The listing builds one solid part. Answer for the finished solid, in the listing's coordinates (mm). A direction names the side the tool comes from. Give positions to 0.01 mm unless a question says otherwise; leave off trailing zeros. Loops run counter-clockwise (first coordinate to the right, second up) from the corner with the lowest first, then second, coordinate; pieces in that order, holes last. Notation, with made-up numbers: M -6,57 L 37,57 A21 cw 37,81 Z; hole C 51,2 d2. An arc over 180 degrees is marked long. Return JSON: item names as keys, results as strings.
from build123d import *

# Parameters (mm, degrees)
BOSS_EXTRUDE1_DEPTH = 100
SKETCH4_W           = 60
SKETCH4_H           = 100
CUT_EXTRUDE2_DEPTH  = 71


with BuildPart() as part:
    # Sketch1 → Boss-Extrude1 (new body)
    with BuildSketch(Plane(origin=(0, 0, 0), x_dir=(0, 0, -1), z_dir=(1, 0, 0))):
        Polygon((-75, 0), (75, 0), (15, 70), (-45, 70), align=None)
        Polygon((-38.40603842, 60), (10.400650775, 60), (53.257793632, 10), (-59.834609849, 10), align=None, mode=Mode.SUBTRACT)
    extrude(amount=BOSS_EXTRUDE1_DEPTH)

    # Sketch4 → Cut-Extrude2 (cut, through all)
    with BuildSketch(Plane(origin=(0, 70, 0), x_dir=(1, 0, 0), z_dir=(0, 1, 0))):
        with Locations((50, 25.697233142)):
            Rectangle(SKETCH4_W, SKETCH4_H)
    extrude(amount=-CUT_EXTRUDE2_DEPTH, mode=Mode.SUBTRACT)


solid = part.part
(1) Determine the mould class of faces 4 (the flat face through (100, 9, 6)), 5 (the flat face through (49, 10, 28)), 6 (the flat face through (50, 5, 24.303)) for opening direction X: released by +X, released by -X, zero draft, split by the parting line, or undercut.
Values follow:
{"face 4": "released by +X", "face 5": "zero draft", "face 6": "undercut"}
(2) The part is cut by section D-D (y = 34.5). Determine the outline of the cut face in (x, z).
Values follow:
{"outline": "M 0,-45.43 L 20,-45.43 L 20,-32.26 L 0,-32.26 Z; M 0,49.33 L 100,49.33 L 100,60.21 L 0,60.21 Z; M 80,-45.43 L 100,-45.43 L 100,-32.26 L 80,-32.26 Z"}
(3) Straight lines are drawn through the part: line 1 along Y through (x, z) = (12.5, 21); line 2 along X through (y, z) = (21, -56); line 3 along Z through (x, y) = (6.5, 52.5). For each, find the intervals that lie inside material, in ascending order.
Values follow:
{"line 1": "0 to 10, 60 to 70", "line 2": "0 to 20, 80 to 100", "line 3": "-30 to -16.83, 41.62 to 52.5"}
(4) A tool of negligible diameter and unlimited length cuts with its end or side. For faces 1 (the flat face through (80, 35.2, -32.5)), 2 (the flat face through (49.3, 34.65, 49.27)), 3 (the flat face through (49, 35, 60)), from which of +Z, -Z, +X, -X, +Y, -Y can it reach the whole face along a straight path? Write none if from no direction.
Values follow:
{"face 1": "-Z, +Y, -Y", "face 2": "+X, -X", "face 3": "+Z, +X, -X, +Y"}
(5) The part is cut by section B-B (z = 16.5). Determine the outline of the cut face in (x, y), and give its area (3 significant figures).
Values follow:
{"outline": "M 0,0 L 20,0 L 20,10 L 0,10 Z; M 0,60 L 20,60 L 20,70 L 0,70 Z; M 80,0 L 100,0 L 100,10 L 80,10 Z; M 80,60 L 100,60 L 100,70 L 80,70 Z", "area": "800 mm²"}
(6) The part is cut by section A-A (z = 33). Determine the outline of the cut face in (x, y), and give its area (3 significant figures).
Values follow:
{"outline": "M 0,0 L 100,0 L 100,10 L 0,10 Z; M 0,60 L 100,60 L 100,70 L 0,70 Z", "area": "2,000 mm²"}
(7) The part is cut by section C-C (x = 14.5). Determine the outline of the cut face in (y, z).
Values follow:
{"outline": "M 0,-75 L 70,-15 L 70,45 L 0,75 Z; hole M 10,-53.26 L 60,-10.4 L 60,38.41 L 10,59.83 Z"}
(8) Given pin 1 (11 mm diameter, centred on x = 42, y = 6.5, fed in from -Z); pin 2 (2 mm diameter, centred on x = 58.5, y = 29.5, fed in from +Z); pin 3 (14.5 mm diameter, centred on x = 46, z = 20.5, fed in from -Y); pin 4 (2 mm diameter, centred on x = 21.5, z = -53.5, fed in from -Y), each flat-ended and moving along its own axis, determine where each tip first touches the part or whether it passes through.
Values follow:
{"pin 1": "z = 24.3", "pin 2": "z = 62.79", "pin 3": "y = 0", "pin 4": "through"}
